The model under review builds one solid part; all positions refer to its coordinate system, in mm. Face numbers are marked on the shaded views. A direction names the side the tool comes from. Give positions to 0.01 mm unless a question says otherwise; leave off trailing zeros. Write each loop counter-clockwise with the first axis right and the second up, starting at its lowest first coordinate (ties: lowest second). Pieces come first, ordered by that corner, then holes. Notation, with made-up numbers: (8.5, -8.75) - (27.5, -8.75) arc R16 cw to (27.5, -0.75) - close; hole circle Ø7 at (0, 71.5). An arc over 180 degrees is marked (long way). Write item = value, one per line.
```python
from build123d import *

# Parameters (mm, degrees)
PAD008_DEPTH         = 50
SKETCH025_W          = 40.7
SKETCH025_H          = 40.7
POCKET016_DEPTH      = 10.5
POCKET017_DEPTH      = 11
POCKET018_DEPTH      = 7
POCKET019_DEPTH      = 7
SKETCH029_W          = 41
SKETCH029_H          = 7.5
POCKET020_DEPTH      = 8
POCKET021_DEPTH      = 100.001
SKETCH031_R          = 1
POCKET022_DEPTH      = 5
SKETCH032_R          = 1
SKETCH032_W          = 19
SKETCH032_H          = 6.5
POCKET023_DEPTH      = 10
SKETCH034_R          = 1.55
POCKET024_DEPTH      = 23.001
SKETCH036_R          = 5
POCKET025_DEPTH      = 2
FILLET013_R          = 2
SKETCH037_W          = 72
SKETCH037_H          = 72
POCKET026_DEPTH      = 2.5
POCKET026_DEPTH_BACK = 11
SKETCH038_W          = 80
SKETCH038_H          = 80
POCKET027_DEPTH      = 2.5


with BuildPart() as part:
    # Sketch024 → Pad008 (new body, symmetric)
    with BuildSketch(Plane.YZ):
        with BuildLine():
            ThreePointArc((-76.283394, 0), (-73.65331, -8.9261), (-66.603462, -15))
            Line((-66.603462, -15), (66.603462, -15))
            ThreePointArc((66.603462, -15), (73.65331, -8.9261), (76.283394, 0))
            Line((-76.283394, 0), (76.283394, 0))
        make_face()
    extrude(amount=PAD008_DEPTH, both=True)

    # Sketch025 (on Face4 of Pad008) → Pocket016 (cut)
    with BuildSketch(Plane(origin=(0, 0, 0), x_dir=(0, -1, 0), z_dir=(0, 0, 1))):
        with Locations((-40.65, -28.15)):
            Rectangle(SKETCH025_W, SKETCH025_H)
        with Locations((-40.65, 28.15)):
            Rectangle(SKETCH025_W, SKETCH025_H)
        Polygon((-66, 3.8), (-16.65, 3.8), (-16.65, 42), (16.35, 42), (16.35, 3.8), (20, 3.8), (20, 42.5), (61, 42.5), (61, -42.5), (20, -42.5), (20, -3.8), (16.35, -3.8), (16.35, -42), (-16.65, -42), (-16.65, -3.8), (-66, -3.8), align=None)
    extrude(amount=-POCKET016_DEPTH, mode=Mode.SUBTRACT)

    # Sketch026 (on Face2 of Pocket016) → Pocket017 (cut)
    with BuildSketch(Plane(origin=(0, 0, 0), x_dir=(0, -1, 0), z_dir=(0, 0, 1))):
        Polygon((-71, 23), (-66, 23), (-66, 21), (-61, 21), (-61, -21), (-66, -21), (-66, -23), (-71, -23), align=None)
        Polygon((66, 23), (71, 23), (71, -23), (66, -23), (66, -7.5), (61, -7.5), (61, 7.5), (66, 7.5), align=None)
    extrude(amount=-POCKET017_DEPTH, mode=Mode.SUBTRACT)

    # Sketch027 (on Face41 of Pocket017) → Pocket018 (cut)
    with BuildSketch(Plane(origin=(0, 71, 0), x_dir=(0, 0, -1), z_dir=(0, -1, 0))):
        with BuildLine():
            ThreePointArc((0, 4.5), (8.5, 13), (0, 21.5))
            Line((0, 21.5), (0, 4.5))
        make_face()
        with BuildLine():
            ThreePointArc((0, -21.5), (8.5, -13), (0, -4.5))
            Line((0, -4.5), (0, -21.5))
        make_face()
    extrude(amount=-POCKET018_DEPTH, mode=Mode.SUBTRACT)

    # Sketch028 (on Face22 of Pocket017) → Pocket019 (cut)
    with BuildSketch(Plane.ZX.offset(-71)):
        with BuildLine():
            ThreePointArc((0, 21.5), (-8.5, 13), (0, 4.5))
            Line((0, 21.5), (0, 4.5))
        make_face()
        with BuildLine():
            ThreePointArc((0, -4.5), (-8.5, -13), (0, -21.5))
            Line((0, -4.5), (0, -21.5))
        make_face()
    extrude(amount=-POCKET019_DEPTH, mode=Mode.SUBTRACT)

    # Sketch029 (on Face2 of Pocket016) → Pocket020 (cut)
    with BuildSketch(Plane(origin=(0, 0, 0), x_dir=(0, -1, 0), z_dir=(0, 0, 1))):
        with Locations((40.5, 46.25)):
            Rectangle(SKETCH029_W, SKETCH029_H)
        with Locations((40.5, -46.25)):
            Rectangle(SKETCH029_W, SKETCH029_H)
    extrude(amount=-POCKET020_DEPTH, mode=Mode.SUBTRACT)

    # Sketch030 → Pocket021 (cut, through all)
    with BuildSketch(Plane.YZ.offset(50)):
        with BuildLine():
            ThreePointArc((44, 0), (51, -7), (58, 0))
            Line((44, 0), (58, 0))
        make_face()
    extrude(amount=-POCKET021_DEPTH, mode=Mode.SUBTRACT)

    # Sketch031 → Pocket022 (cut)
    with BuildSketch(Plane.YZ.offset(50)):
        with Locations((31, -7)):
            Circle(SKETCH031_R)
        with Locations((44, -8)):
            Circle(SKETCH031_R)
    extrude(amount=-POCKET022_DEPTH, mode=Mode.SUBTRACT)

    # Sketch032 → Pocket023 (cut)
    with BuildSketch(Plane(origin=(-50, 0, 0), x_dir=(0, 1, 0), z_dir=(-1, 0, 0))):
        with Locations((31, 7)):
            Circle(SKETCH032_R)
        with Locations((44, 8)):
            Circle(SKETCH032_R)
        with Locations((0, 3.25)):
            Rectangle(SKETCH032_W, SKETCH032_H)
    extrude(amount=-POCKET023_DEPTH, mode=Mode.SUBTRACT)

    # Sketch034 → Pocket024 (cut, through all)
    with BuildSketch(Plane(origin=(0, 0, 8), x_dir=(0, -1, 0), z_dir=(0, 0, 1))):
        with Locations((42, 46.25)):
            Circle(SKETCH034_R)
        with Locations((42, -46.25)):
            Circle(SKETCH034_R)
        with Locations((-16, -46.25)):
            Circle(SKETCH034_R)
        with Locations((0, 46.25)):
            Circle(SKETCH034_R)
        with Locations((-65, 46.25)):
            Circle(SKETCH034_R)
        with Locations((-65, -46.25)):
            Circle(SKETCH034_R)
    extrude(amount=-POCKET024_DEPTH, mode=Mode.SUBTRACT)

    # Sketch036 → Pocket025 (cut)
    with BuildSketch(Plane.YX.offset(15)):
        with Locations((-42, 46.25)):
            Circle(SKETCH036_R)
        with Locations((-42, -46.25)):
            Circle(SKETCH036_R)
        with Locations((16, -46.25)):
            Circle(SKETCH036_R)
        with Locations((0, 46.25)):
            Circle(SKETCH036_R)
        with Locations((65, 46.25)):
            Circle(SKETCH036_R)
        with Locations((65, -46.25)):
            Circle(SKETCH036_R)
    extrude(amount=-POCKET025_DEPTH, mode=Mode.SUBTRACT)

    # Fillet013
    fillet013_edges = [part.edges().sort_by_distance(p)[0] for p in [
        (46.25, -61, -8),
        (46.25, -20, -8),
        (-46.25, -20, -8),
        (-46.25, -61, -8),
    ]]
    fillet(fillet013_edges, radius=FILLET013_R)

    # Sketch037 (on Face69 of Fillet013) → Pocket026 (cut, two sides)
    with BuildSketch(Plane(origin=(0, 0, -10.5), x_dir=(0, -1, 0), z_dir=(0, 0, 1))) as pocket026_sk:
        with Locations((24, 0)):
            Rectangle(SKETCH037_W, SKETCH037_H)
    extrude(amount=-POCKET026_DEPTH, mode=Mode.SUBTRACT)
    extrude(pocket026_sk.sketch, amount=POCKET026_DEPTH_BACK, mode=Mode.SUBTRACT)

    # Sketch038 (on Face5 of Pocket026) → Pocket027 (cut)
    with BuildSketch(Plane.YX.offset(15)):
        with Locations((-24, 0)):
            Rectangle(SKETCH038_W, SKETCH038_H)
    extrude(amount=-POCKET027_DEPTH, mode=Mode.SUBTRACT)


solid = part.part
```
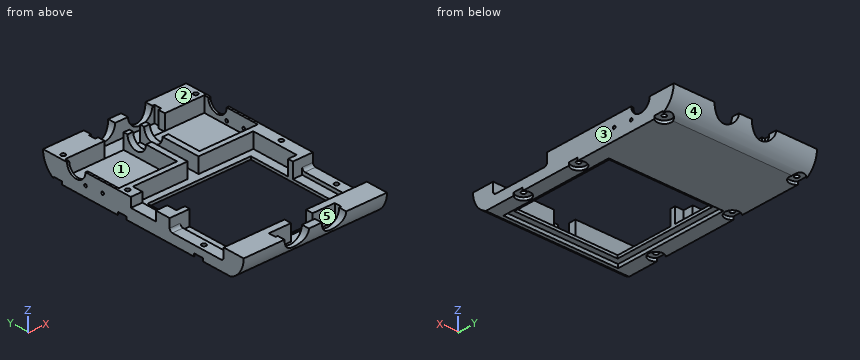
1. Machinability: for the marked faces 1 and 2, which of the approach directions +Z, -Z, +X, -X, +Y, -Y give a long, thin tool a straight path to every point of the face, cutting with its end or side? Answer none if there is none.
Findings below:
face_1 = +Z
face_2 = +Z, +X, -X, +Y, -Y
2. Take a section at B-B on x = 27. Give the boundary of the cut face in (y, z), and give its area (3 significant figures).
Findings below:
outline = (-76.28, 0) arc R16.46 ccw to (-66.6, -15) - (-64, -15) - (-64, -12.5) - (-60, -12.5) - (-60, -10.5) - (-61, -10.5) - (-61, 0) - close; (12, -12.5) - (16, -12.5) - (16, -15) - (66.6, -15) arc R16.46 ccw to (76.28, 0) - (61, 0) - (61, -10.5) - (20.3, -10.5) - (20.3, 0) - (16.65, 0) - (16.65, -10.5) - (12, -10.5) - close
area = 620 mm²
3. Insertion check: P1, Ø5, axis at x = 46.25, y = 65, coming from the -Z side; P2, Ø1.2, axis at y = 44, z = -8, coming from the +X side; P3, Ø3, axis at x = 40, z = -3, coming from the -Y side. Each pin has a flat end and moves straight along its axis. Give the tip position at first contact, or say it passes through.
Findings below:
P1 = -13
P2 = 7.8
P3 = -76.21
4. Take a section at D-D on y = 51. Give the boundary of the cut face in (x, z).
Findings below:
outline = (-50, -15) - (50, -15) - (50, -7) - (48.5, -7) - (48.5, -10.5) - (7.8, -10.5) - (7.8, -7) - (3.8, -7) - (3.8, -10.5) - (-3.8, -10.5) - (-3.8, -7) - (-7.8, -7) - (-7.8, -10.5) - (-48.5, -10.5) - (-48.5, -7) - (-50, -7) - close
5. Take a section at C-C on y = -42. Give the boundary of the cut face in (x, z).
Findings below:
outline = (-50, -13) - (-47.8, -13) - (-47.8, -8) - (-50, -8) - close; (-44.7, -13) - (-41.25, -13) - (-41.25, -15) - (-40, -15) - (-40, -12.5) - (-36, -12.5) - (-36, -10.5) - (-42.5, -10.5) - (-42.5, -8) - (-44.7, -8) - close; (36, -12.5) - (40, -12.5) - (40, -15) - (41.25, -15) - (41.25, -13) - (44.7, -13) - (44.7, -8) - (42.5, -8) - (42.5, -10.5) - (36, -10.5) - close; (47.8, -13) - (50, -13) - (50, -8) - (47.8, -8) - close
6. Draft analysis for pull direction Y (two halves, no side actions). For the marked faces 3, 4 and 5, state which applies: +Y half, -Y half, draft (parallel to the pull), parting line (faces both ways), or undercut.
Findings below:
face_3 = draft
face_4 = +Y half
face_5 = undercut
7. For line 1 (X direction, y = 21, z = -0.75); line 2 (X direction, y = 11.5, z = -2.75); line 3 (X direction, y = -19, z = -2.5), list the stretches that pass through material, from the lowest coordinate up. Write a range as from..to.
Findings below:
line_1 = -50..-48.5, -7.8..-3.8, 3.8..7.8, 48.5..50
line_2 = -50..-42, 42..50
line_3 = -50..-36, 36..50
8. Take a section at A-A on y = 0. Give the boundary of the cut face in (x, z).
Findings below:
outline = (-50, -15) - (-40, -15) - (-40, -12.5) - (-36, -12.5) - (-36, -10.5) - (-42, -10.5) - (-42, -6.5) - (-50, -6.5) - close; (36, -12.5) - (40, -12.5) - (40, -15) - (41.25, -15) - (41.25, -13) - (44.7, -13) - (44.7, 0) - (42, 0) - (42, -10.5) - (36, -10.5) - close; (47.8, -13) - (50, -13) - (50, 0) - (47.8, 0) - close
